from build123d import *

# Parameters (mm, degrees)
SKETCH_3_R      = 1.5
SKETCH_3_R_2    = 2
EXTRUDE_1_DEPTH = 4


with BuildPart() as part:
    # 草图3 → 凸台-拉伸1 (new body)
    with BuildSketch(Plane.XY):
        Polygon((-46.5, 5.009783315), (-37.5, 5.009783315), (-37.5, 14.509783315), (37.5, 14.509783315), (37.5, 5.009783315), (46.5, 5.009783315), (46.5, -19.990216685), (44, -19.990216685), (44, -18.490216685), (41.4, -18.490216685), (41.4, -19.990216685), (38.4, -19.990216685), (38.4, -22.990216685), (41.4, -22.990216685), (41.4, -24.490216685), (44, -24.490216685), (44, -22.990216685), (46.5, -22.990216685), (46.5, -32.990216685), (49.5, -32.990216685), (49.5, -40.990216685), (46.5, -40.990216685), (46.5, -99.795048798), (28.5, -301.990216685), (28.5, -330.990216685), (31.5, -330.990216685), (31.5, -338.990216685), (28.5, -338.990216685), (28.5, -348.990216685), (26, -348.990216685), (26, -347.490216685), (23.4, -347.490216685), (23.4, -348.990216685), (20.4, -348.990216685), (20.4, -351.990216685), (23.4, -351.990216685), (23.4, -353.490216685), (26, -353.490216685), (26, -351.990216685), (28.5, -351.990216685), (28.5, -365.490216685), (-28.5, -365.490216685), (-28.5, -351.990216685), (-26, -351.990216685), (-26, -353.490216685), (-23.4, -353.490216685), (-23.4, -351.990216685), (-20.4, -351.990216685), (-20.4, -348.990216685), (-23.4, -348.990216685), (-23.4, -347.490216685), (-26, -347.490216685), (-26, -348.990216685), (-28.5, -348.990216685), (-28.5, -338.990216685), (-31.5, -338.990216685), (-31.5, -330.990216685), (-28.5, -330.990216685), (-28.5, -301.990216685), (-46.5, -99.795048798), (-46.5, -40.990216685), (-49.5, -40.990216685), (-49.5, -32.990216685), (-46.5, -32.990216685), (-46.5, -22.990216685), (-44, -22.990216685), (-44, -24.490216685), (-41.4, -24.490216685), (-41.4, -22.990216685), (-38.4, -22.990216685), (-38.4, -19.990216685), (-41.4, -19.990216685), (-41.4, -18.490216685), (-44, -18.490216685), (-44, -19.990216685), (-46.5, -19.990216685), align=None)
        with Locations((-31.5, -0.990216685)):
            Circle(SKETCH_3_R, mode=Mode.SUBTRACT)
        with Locations((0, 10.509783315)):
            Circle(SKETCH_3_R_2, mode=Mode.SUBTRACT)
        with Locations(Location((31.5, -0.990216685, 0), (0, 0, 180))):
            Circle(SKETCH_3_R, mode=Mode.SUBTRACT)
        with Locations((0, -361.990216685)):
            Circle(SKETCH_3_R, mode=Mode.SUBTRACT)
        with Locations((-20.4, -356.990216685)):
            Circle(SKETCH_3_R, mode=Mode.SUBTRACT)
        with Locations(Location((20.4, -356.990216685, 0), (0, 0, 180))):
            Circle(SKETCH_3_R, mode=Mode.SUBTRACT)
        with BuildLine():
            Line((-17.023193691, -146.328074808), (-17.023193691, -46.328074808))
            ThreePointArc((-17.023193691, -46.328074808), (0, -29.304881117), (17.023193691, -46.328074808))
            Line((17.023193691, -46.328074808), (17.023193691, -146.328074808))
            ThreePointArc((17.023193691, -146.328074808), (0, -163.351268499), (-17.023193691, -146.328074808))
        make_face(mode=Mode.SUBTRACT)
        with BuildLine():
            Line((-15, -207.652358563), (-15, -271.328074808))
            ThreePointArc((-15, -271.328074808), (0, -286.328074808), (15, -271.328074808))
            Line((15, -271.328074808), (15, -207.652358563))
            ThreePointArc((15, -207.652358563), (0, -192.652358563), (-15, -207.652358563))
        make_face(mode=Mode.SUBTRACT)
    extrude(amount=EXTRUDE_1_DEPTH)


solid = part.part
Input: part model. Units: mm. Frame: model coordinates. A direction names the side the tool comes from. Coordinates: 2 decimals unless noted, no trailing zeros. Order: outer loops, then holes, each group sorted by start corner. A loop starts at its lowest first (then second) coordinate and runs counter-clockwise, first axis right, second up. Notation, with made-up numbers: M 56.25,39 L 77.25,39 A5 cw 77.25,45 Z; hole C -37,15 d9. An arc over 180 degrees is marked long. One line per question, with ' | ' between items.
Item 1: Reachability of faces 1 (the cylindrical face through (-0.33, -286.324, 1.972)), 2 (the flat face through (1, -173, 0)), 3 (the flat face through (-37.374, -202.308, 1.972)) from +Z, -Z, +X, -X, +Y, -Y: full face, straight path, thin tool, end or side. Return the list, or none.
Geometry results:
face 1: +Z, -Z | face 2: -Z, +X, -X, +Y, -Y | face 3: +Z, -Z, -X
Item 2: Section D-D (y = -316.5). Output: boundary loops of the cut face in (x, z).
Geometry results:
outline: M -28.5,0 L 28.5,0 L 28.5,4 L -28.5,4 Z
Item 3: Pin query (flat end, axial travel): pin 1 (0.9 mm diameter, centred on x = -30, z = 3, fed in from -Y); pin 2 (1.5 mm diameter, centred on x = 48.5, z = 3, fed in from -Y); pin 3 (1.2 mm diameter, centred on y = -19, z = 2.5, fed in from +X). Return the tip coordinate at first contact, or that it passes through.
Geometry results:
pin 1: stops at y = -338.99 | pin 2: stops at y = -40.99 | pin 3: stops at x = 46.5
Item 4: Ray query, line 1 along Y through (x, z) = (0, 3.15); line 2 along Y through (x, z) = (20, 2.35); line 3 along Y through (x, z) = (-27, 0.7). Return the intervals inside material, ascending.
Geometry results:
line 1: y = -365.49 to -363.49, -360.49 to -286.33, -192.65 to -163.35, -29.3 to 8.51, 12.51 to 14.51 | line 2: y = -365.49 to -358.44, -355.54 to 14.51 | line 3: y = -365.49 to -351.99, -348.99 to 14.51
Item 5: Draft query along Y for faces 4 (the cylindrical face through (0.374, -163.347, 1.972)), 5 (the cylindrical face through (0.33, -192.656, 1.972)), 6 (the flat face through (1, -173, 4)). Return one class per face: released by +Y, released by -Y, zero draft, split by the parting line, or undercut.
Geometry results:
face 4: undercut | face 5: undercut | face 6: zero draft
Item 6: Section A-A (y = -198). Output: boundary loops of the cut face in (x, z).
Geometry results:
outline: M -37.76,0 L -11.48,0 L -11.48,4 L -37.76,4 Z; M 11.48,0 L 37.76,0 L 37.76,4 L 11.48,4 Z
Item 7: Section B-B (y = -255.5). Output: boundary loops of the cut face in (x, z).
Geometry results:
outline: M -32.64,0 L -15,0 L -15,4 L -32.64,4 Z; M 15,0 L 32.64,0 L 32.64,4 L 15,4 Z
Item 8: Section C-C (z = 3.1). Give the number of separate pieces and of enclosed holes in the cut face, then the cut area to 3 significant figures.
Geometry results:
separate pieces: 1 | enclosed holes: 8 | area: 22,200 mm^2
